Could you check a few things on this model? Use its own coordinates, in mm. Face numbers are marked on the shaded views. A direction names the side the tool comes from. Give positions to 0.01 mm unless a question says otherwise; leave off trailing zeros. Loops run counter-clockwise (first coordinate to the right, second up) from the corner with the lowest first, then second, coordinate; pieces in that order, holes last. Notation, with made-up numbers: (68.5, -7.75) - (84.5, -7.75) arc R8 ccw to (84.5, -2.75) - close; hole circle Ø7 at (13.5, -12.75). An arc over 180 degrees is marked (long way). One line per item, written item: value. Start each with the question number.
Q1. For the marked faces 1 and 2, which set-ups out of +Z, -Z, +X, -X, +Y, -Y let a thin tool reach every point of the face, with its end or its side?
Q2. If I drill on line 1 (Y direction, x = -0.8, z = 4.5); line 2 (Z direction, x = -0.05, y = 5.5); line 3 (Z direction, x = 1.85, y = 3.75), over which ranges is the centre line in solid material (lowest first)? Write a range as from..to.
Q3. I'm going to push flat-ended pins straight in: P1, Ø1.5, axis at x = -1.5, z = -4.5, coming from the -Y side; P2, Ø4, axis at y = 4.49, z = 4.49, coming from the +X side. Where does each tip first touch, or does it pass through?
Q4. I want a section at C-C (x = -0.7). Please give me the cut outline in (y, z), then the cut area to 3 significant figures.
Q5. If we mould it in two halves opening along Z, with no side actions, what happens to the marked faces 3, 4 and 5? For each: released by +Z, released by -Z, zero draft, split by the parting line, or undercut.
Q6. I want a section at A-A (y = 0). Please give me the cut outline in (x, z).
Q7. I want a section at D-D (y = -5.25). Count the separate pieces of the cut face and the enclosed holes in it, then the cut area to 3 significant figures.
Q8. I want a section at B-B (z = 0). Please give me the cut outline in (x, y).
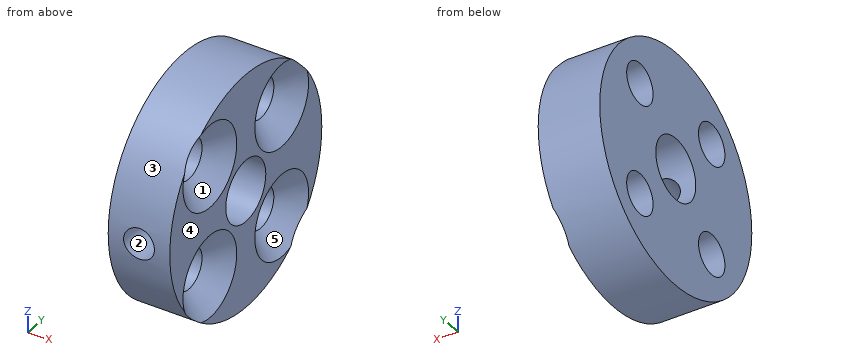
```python
from build123d import *

# Parameters (mm, degrees)
F0_R           = 9.5
F0_R_2         = 2.5
F1_DEPTH       = 2.5
F3_R           = 1.25
F4_DEPTH       = 9.501
F5_D           = 3.3
F5_CSINK_D     = 6.72
F5_CSINK_ANGLE = 90


with BuildPart() as f1:
    # F0 (on Right) → F1 (new body, symmetric)
    with BuildSketch(Plane.YZ):
        Circle(F0_R)
        Circle(F0_R_2, mode=Mode.SUBTRACT)
    extrude(amount=F1_DEPTH, both=True)

    # F3 (on Front) → F4 (cut, through all)
    with BuildSketch(Plane.XZ):
        Circle(F3_R)
    extrude(amount=F4_DEPTH, mode=Mode.SUBTRACT)

    # F5 (through all)
    with Locations(Plane.YZ.offset(2.5)):
        with Locations((-4.4901280605, 4.4901280605), (4.4901280605, 4.4901280605), (4.4901280605, -4.4901280605), (-4.4901280605, -4.4901280605)):
            CounterSinkHole(F5_D / 2, F5_CSINK_D / 2, counter_sink_angle=F5_CSINK_ANGLE)


solid = f1.part
```
Worked answers:
1. face 1: +X
1. face 2: -Y
2. line 1: y = -8.37..-6.14, -2.84..2.84, 6.14..8.37
2. line 2: z = -7.75..-5.79, -3.19..3.19, 5.79..7.75
2. line 3: z = -8.73..-7.1, -1.88..1.88, 7.1..8.73
3. P1: stops at y = -8.73
3. P2: stops at x = 1.14
4. outline: (-9.44, -1.04) arc R9.5 ccw (long way) to (-9.44, 1.04) - (-2.28, 1.04) arc R2.5 cw (long way) to (-2.28, -1.04) - close; hole circle Ø3.3 at (-4.49, -4.49); hole circle Ø3.3 at (-4.49, 4.49); hole circle Ø3.3 at (4.49, -4.49); hole circle Ø3.3 at (4.49, 4.49)
4. area: 215 mm²
5. face 3: split by the parting line
5. face 4: zero draft
5. face 5: undercut
6. outline: (-2.5, -9.5) - (2.5, -9.5) - (2.5, -2.5) - (-2.5, -2.5) - close; (-2.5, 2.5) - (2.5, 2.5) - (2.5, 9.5) - (-2.5, 9.5) - close
7. separate pieces: 3
7. enclosed holes: 1
7. area: 38.7 mm²
8. outline: (-2.5, -9.5) - (-1.25, -9.5) - (-1.25, -2.5) - (-2.5, -2.5) - close; (-2.5, 2.5) - (2.5, 2.5) - (2.5, 9.5) - (-2.5, 9.5) - close; (1.25, -9.5) - (2.5, -9.5) - (2.5, -2.5) - (1.25, -2.5) - close
